CAD build for the part. Positions are in the model's coordinates, mm. A direction names the side the tool comes from. Give positions to 0.01 mm unless a question says otherwise; leave off trailing zeros. Loops run counter-clockwise (first coordinate to the right, second up) from the corner with the lowest first, then second, coordinate; pieces in that order, holes last.
```python
from build123d import *

# Parameters (mm, degrees)
SKETCH2_W = 72
SKETCH2_H = 36


with BuildPart() as part:
    # Sweep1: sweep along a path in Sketch1
    with BuildLine(Plane.XY) as sweep1_path:
        Line((0, 0), (-50, 0))
        ThreePointArc((-50, 0), (-110, 60), (-50, 120))
        Line((-50, 120), (200, 120))
    # Sketch2 → Sweep1 (sweep)
    with BuildSketch(Plane(origin=(0, 0, 0), x_dir=(0, 0, -1), z_dir=(1, 0, 0))):
        Rectangle(SKETCH2_W, SKETCH2_H)
    sweep(path=sweep1_path.line)


solid = part.part
```
1. Tool access for faces 1 (the face through (0, 0, -1)), 2 (the face through (-25, 18, -1)), 3 (the face through (200, 120, 1)): list every direction of +Z, -Z, +X, -X, +Y, -Y with a clear straight run to the whole face (end or side of a thin tool).
Responses:
face 1: +Z, -Z, +X, -Y
face 2: +Z, -Z, +X
face 3: +Z, -Z, +X, +Y, -Y
2. Saw through at A-A, the plane z = 13. List the corners of the cut face in (x, y).
Responses:
outline: (-50, -18) - (0, -18) - (0, 18) - (-50, 18) arc R42 cw to (-50, 102) - (200, 102) - (200, 138) - (-50, 138) arc R78 ccw to start
3. Drop flat-ended pins along their axis: pin 1 (8 mm diameter, centred on y = 34.5, z = 16, fed in from +X); pin 2 (4 mm diameter, centred on y = 61.5, z = 19.5, fed in from -X); pin 3 (18 mm diameter, centred on y = 7.5, z = 7.5, fed in from +X). Give the stop position or say it passes through.
Responses:
pin 1: stops at x = -79.9
pin 2: stops at x = -128
pin 3: stops at x = 0
4. Saw through at B-B, the plane x = -72.5. List the corners of the cut face in (y, z), and give its area (3 significant figures).
Responses:
outline: (-14.68, -36) - (24.54, -36) - (24.54, 36) - (-14.68, 36) - close; (95.46, -36) - (134.68, -36) - (134.68, 36) - (95.46, 36) - close
area: 5,650 mm2
5. Saw through at C-C, the plane x = 98. List the corners of the cut face in (y, z).
Responses:
outline: (102, -36) - (138, -36) - (138, 36) - (102, 36) - close
6. Probe line 1 along Y through (x, z) = (-18, 29.5); line 2 along Y through (x, z) = (28, 18.5); line 3 along X through (y, z) = (39.5, 1.5). List the from-to ranges inside material, lowest first.
Responses:
line 1: y = -18 to 18, 102 to 138
line 2: y = 102 to 138
line 3: x = -125.26 to -86.66
7. Saw through at D-D, the plane y = 60. List the corners of the cut face in (x, z).
Responses:
outline: (-128, -36) - (-92, -36) - (-92, 36) - (-128, 36) - close
8. Pull direction Y, two halves, no side cores. Call faces 4 (the face through (11, 106, -36)), 5 (the face through (-127.98, 58.28, -0.5)), 6 (the face through (-91.99, 59.08, 0.5)): released by +Y, released by -Y, zero draft, split by the parting line, or undercut.
Responses:
face 4: zero draft
face 5: split by the parting line
face 6: undercut
